Model file for the job. Use its own axes, mm. Face numbers are marked on the shaded views. Round coordinates to 2 decimals unless told otherwise and drop trailing zeros. Loops run counter-clockwise (first coordinate to the right, second up) from the corner with the lowest first, then second, coordinate; pieces in that order, holes last. Notation, with made-up numbers: (-26.75, -38.75) - (0.25, -38.75) arc R25 cw to (0.25, -0.75) - close; hole circle Ø9 at (88.25, 6). An arc over 180 degrees is marked (long way). Answer as a JSON object with one key per item and string values.
from build123d import *

# Parameters (mm, degrees)
SKETCH_R      = 48
SKETCH_R_2    = 42
PAD_DEPTH     = 3
SKETCH001_R   = 45.5
SKETCH001_R_2 = 42
PAD001_DEPTH  = 5.5
CHAMFER_SIZE  = 1
SKETCH002_R   = 5
POCKET_DEPTH  = 5.501


with BuildPart() as part:
    # Sketch → Pad (new body)
    with BuildSketch(Plane.XY):
        Circle(SKETCH_R)
        Circle(SKETCH_R_2, mode=Mode.SUBTRACT)
    extrude(amount=PAD_DEPTH)

    # Sketch001 (on Face4 of Pad) → Pad001 (join)
    with BuildSketch(Plane.XY.offset(3)):
        Circle(SKETCH001_R)
        Circle(SKETCH001_R_2, mode=Mode.SUBTRACT)
    extrude(amount=PAD001_DEPTH)

    # Chamfer
    chamfer_edges = [part.edges().sort_by_distance(p)[0] for p in [
        (-42, 0, 8.5),
    ]]
    chamfer(chamfer_edges, length=CHAMFER_SIZE)

    # Sketch002 → Pocket (cut, through all)
    with BuildSketch(Plane.XY.offset(3)):
        with Locations((31.496593, 37.536178)):
            Circle(SKETCH002_R)
        with Locations((48.25558, 8.508761)):
            Circle(SKETCH002_R)
        with Locations((42.435245, -24.5)):
            Circle(SKETCH002_R)
        with Locations((16.758987, -46.044938)):
            Circle(SKETCH002_R)
        with Locations((-16.758987, -46.044938)):
            Circle(SKETCH002_R)
        with Locations((-42.435245, -24.5)):
            Circle(SKETCH002_R)
        with Locations((-48.25558, 8.508761)):
            Circle(SKETCH002_R)
        with Locations((-31.496593, 37.536178)):
            Circle(SKETCH002_R)
        with Locations((0, 49)):
            Circle(SKETCH002_R)
    extrude(amount=POCKET_DEPTH, mode=Mode.SUBTRACT)


solid = part.part
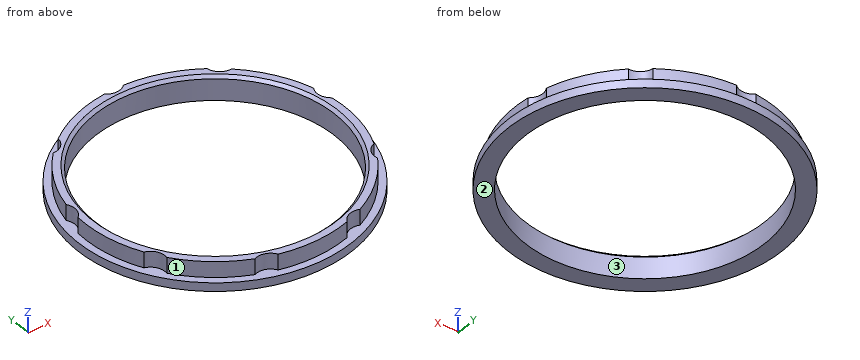
1) Slice it at C-C on y = 0. List the corners of the cut face in (x, z), then the cut area to 3 significant figures.
Values follow:
{"outline": "(-48, 0) - (-42, 0) - (-42, 7.5) - (-43, 8.5) - (-45.5, 8.5) - (-45.5, 3) - (-48, 3) - close; (42, 0) - (48, 0) - (48, 3) - (45.5, 3) - (45.5, 8.5) - (43, 8.5) - (42, 7.5) - close", "area": "73.5 mm²"}
2) Two-plate mould, pull along Y, no slides. Class the marked faces 1, 2 and 3: pulls with the +Y half, pulls with the -Y half, needs draft (parallel to the pull), parting line crosses it, or undercut.
Values follow:
{"face 1": "pulls with the -Y half", "face 2": "needs draft", "face 3": "undercut"}
3) Slice it at B-B on z = 5.75. List the corners of the cut face in (x, y).
Values follow:
{"outline": "(-45.28, 4.49) arc R45.5 ccw to (-41.01, -19.71) arc R5 cw to (-37.57, -25.66) arc R45.5 ccw to (-18.75, -41.46) arc R5 cw to (-12.29, -43.81) arc R45.5 ccw to (12.29, -43.81) arc R5 cw to (18.75, -41.46) arc R45.5 ccw to (37.57, -25.66) arc R5 cw to (41.01, -19.71) arc R45.5 ccw to (45.28, 4.49) arc R5 cw to (44.08, 11.26) arc R45.5 ccw to (31.8, 32.55) arc R5 cw to (26.53, 36.97) arc R45.5 ccw to (3.44, 45.37) arc R5 cw to (-3.44, 45.37) arc R45.5 ccw to (-26.53, 36.97) arc R5 cw to (-31.8, 32.55) arc R45.5 ccw to (-44.08, 11.26) arc R5 cw to start; hole circle Ø84 at (0, 0)"}
4) Slice it at A-A on x = 0. List the corners of the cut face in (y, z), then the cut area to 4 significant figures.
Values follow:
{"outline": "(-48, 0) - (-42, 0) - (-42, 7.5) - (-43, 8.5) - (-45.5, 8.5) - (-45.5, 3) - (-48, 3) - close; (42, 0) - (48, 0) - (48, 3) - (44, 3) - (44, 8.5) - (43, 8.5) - (42, 7.5) - close", "area": "65.25 mm²"}
5) Probe probe 1 along Y at (x, z) = (0, 4.5); probe 2 along X at (y, z) = (32, 2.75); probe 3 along Y at (x, z) = (-38, 8.25). List the from-to ranges inside material, lowest first.
Values follow:
{"probe 1": "-45.5 to -42, 42 to 44", "probe 2": "-35.78 to -27.2, 27.2 to 35.78", "probe 3": "-22.19 to -19.58, 19.58 to 25.02"}
6) Drop flat-ended pins along their axis: P1, Ø1, axis at y = -7, z = 6.5, coming from the -X side; P2, Ø5, axis at x = -0.5, z = 4, coming from the -Y side; P3, Ø4, axis at y = 8, z = 6.5, coming from the -X side. Give the stop position or say it passes through.
Values follow:
{"P1": "x = -45.03", "P2": "y = -48", "P3": "x = -43.93"}
